Input: part model. Units: mm. Frame: model coordinates. A direction names the side the tool comes from. Coordinates: 2 decimals unless noted, no trailing zeros. Order: outer loops, then holes, each group sorted by start corner. A loop starts at its lowest first (then second) coordinate and runs counter-clockwise, first axis right, second up. Notation, with made-up numbers: (58, 82.5) - (65, 82.5) arc R10 ccw to (65, 95.5) - close; hole circle Ø11 at (84, -31.5). An arc over 180 degrees is marked (long way). Answer as CSV lines item,"result". Start each with the question number.
Item 1: Section A-A (z = 11). State how many separate pieces and enclosed holes the cut face has, and give its area (3 significant figures).
Item 2: Draft query along Y for faces 1 (the flat face through (-5, 0, 11)), 2 (the flat face through (0, 5, 22)), 3 (the cylindrical face through (-27.58, 14.44, 11.15)), 4 (the cylindrical face through (-24.733, 9.841, 20.521)). Return one class per face: +Y half, -Y half, draft (parallel to the pull), parting line (faces both ways), or undercut.
Item 3: Material intervals for line 1 along X through (y, z) = (3.3, 11); line 2 along Y through (x, z) = (21.5, 20.4); line 3 along Y through (x, z) = (21.5, 14.25), sorted ascending.
Item 4: Section B-B (x = 0). Output: boundary loops of the cut face in (y, z), and give its area (3 significant figures).
Item 5: First-contact query: pin 1 (5.5 mm diameter, centred on x = -21.5, y = 8.5, fed in from -Z); pin 2 (3 mm diameter, centred on y = 12, z = 11.5, fed in from +X); pin 3 (1.5 mm diameter, centred on y = 7.5, z = 5.5, fed in from +X); pin 4 (5 mm diameter, centred on x = -4.5, z = 18.79, fed in from +Y). Flat tips, straight axial feed; report the tip coordinate or a pass-through.
Item 6: Access query for faces 5 (the flat face through (0, 6, 16)), 6 (the flat face through (0, 5, 0)). Directions: +Z, -Z, +X, -X, +Y, -Y. A direction counts if a zero-diameter tool reaches every point of the face in a straight line with its end or side. Return the directions, or none.
Item 7: Section C-C (y = 3.75). Output: boundary loops of the cut face in (x, z).
from build123d import *

# Parameters (mm, degrees)
BOSS_EXTRU_1_DEPTH      = 22
ESQUISSE3_R             = 6.1
ENL_V_MAT_EXTRU_1_DEPTH = 41.902322672
ESQUISSE4_R             = 4.25
ENL_V_MAT_EXTRU_2_DEPTH = 41.902322672
CONG_1_R                = 8.5
ESQUISSE5_R             = 1.5
ENL_V_MAT_EXTRU_3_DEPTH = 39.794329483
ESQUISSE6_R             = 6.25
ESQUISSE6_R_2           = 3.5
BOSS_EXTRU_2_DEPTH      = 3
CONG_2_R                = 1


with BuildPart() as part:
    # Esquisse2 → Boss.-Extru.1 (new body)
    with BuildSketch(Plane.XY):
        Polygon((-30, 0), (30, 0), (30, 17), (13, 17), (13, 6), (-13, 6), (-13, 17), (-30, 17), align=None)
    extrude(amount=BOSS_EXTRU_1_DEPTH)

    # Esquisse3 → Enlèv. mat.-Extru.1 (cut, through all)
    with BuildSketch(Plane.XY.offset(22)):
        with Locations((21.5, 8.5)):
            Circle(ESQUISSE3_R)
        with Locations(Location((-21.5, 8.5, 0), (0, 0, 180))):
            Circle(ESQUISSE3_R)
    extrude(amount=-ENL_V_MAT_EXTRU_1_DEPTH, mode=Mode.SUBTRACT)

    # Esquisse4 → Enlèv. mat.-Extru.2 (cut, through all)
    with BuildSketch(Plane(origin=(0, 0, 0), x_dir=(-1, 0, 0), z_dir=(0, -1, 0))):
        with Locations(Location((0, -11, 0), (0, 0, 90))):
            Circle(ESQUISSE4_R)
    extrude(amount=-ENL_V_MAT_EXTRU_2_DEPTH, mode=Mode.SUBTRACT)

    # Congé1
    cong_1_edges = [part.edges().sort_by_distance(p)[0] for p in [
        (30, 0, 11),
        (30, 17, 11),
        (-30, 0, 11),
        (-30, 17, 11),
    ]]
    fillet(cong_1_edges, radius=CONG_1_R - 0.0001)  # a hair under: the kernel refuses the full size

    # Esquisse5 → Enlèv. mat.-Extru.3 (cut, through all)
    with BuildSketch(Plane(origin=(0, 6, 0), x_dir=(1, 0, 0), z_dir=(0, 1, 0))):
        with Locations(Location((9, -11, 0), (0, 0, 270))):
            Circle(ESQUISSE5_R)
        with Locations(Location((-4.5, -18.794228634, 0), (0, 0, 270))):
            Circle(ESQUISSE5_R)
        with Locations(Location((-4.5, -3.205771366, 0), (0, 0, 270))):
            Circle(ESQUISSE5_R)
    extrude(amount=-ENL_V_MAT_EXTRU_3_DEPTH, mode=Mode.SUBTRACT)

    # Esquisse6 → Boss.-Extru.2 (add)
    # profile 1 of 2: a face of its own
    with BuildSketch(Plane.XY.offset(22)):
        with Locations((21.5, 8.5)):
            Circle(ESQUISSE6_R)
        with Locations((21.5, 8.5)):
            Circle(ESQUISSE6_R_2, mode=Mode.SUBTRACT)
    # profile 2 of 2: a face of its own
    with BuildSketch(Plane.XY.offset(22)):
        with Locations((-21.5, 8.5)):
            Circle(ESQUISSE6_R)
        with Locations(Location((-21.5, 8.5, 0), (0, 0, 180))):
            Circle(ESQUISSE6_R_2, mode=Mode.SUBTRACT)
    extrude(amount=-BOSS_EXTRU_2_DEPTH)

    # Congé2
    cong_2_edges = [part.edges().sort_by_distance(p)[0] for p in [
        (13, 17, 11),
        (-13, 17, 11),
    ]]
    fillet(cong_2_edges, radius=CONG_2_R)


solid = part.part
Determined:
1,separate pieces,"3"
1,enclosed holes,"2"
1,area,"369 mm^2"
2,face 1,"-Y half"
2,face 2,"draft"
2,face 3,"+Y half"
2,face 4,"undercut"
3,line 1,"x = -28.22 to -24.69, -18.31 to -4.25, 4.25 to 7.5, 10.5 to 18.31, 24.69 to 28.22"
3,line 2,"y = 0 to 5, 12 to 17"
3,line 3,"y = 0 to 2.4, 14.6 to 17"
4,outline,"(0, 0) - (6, 0) - (6, 6.75) - (0, 6.75) - close; (0, 15.25) - (6, 15.25) - (6, 22) - (0, 22) - close"
4,area,"81.0 mm^2"
5,pin 1,"passes through"
5,pin 2,"stops at x = 29.76"
5,pin 3,"stops at x = 30"
5,pin 4,"stops at y = 6"
6,face 5,"+Z, -Z, +Y"
6,face 6,"-Z, +X, -X, +Y, -Y"
7,outline,"(-28.55, 0) - (-25.33, 0) - (-25.33, 19) - (-17.67, 19) - (-17.67, 0) - (17.67, 0) - (17.67, 19) - (25.33, 19) - (25.33, 0) - (28.55, 0) - (28.55, 22) - (-28.55, 22) - close; hole circle Ø3 at (-4.5, 3.21); hole circle Ø3 at (-4.5, 18.79); hole circle Ø8.5 at (0, 11); hole circle Ø3 at (9, 11)"
